Geometry check sheet. Reference: the model listing, model coordinates, mm. Give positions to 0.01 mm unless a question says otherwise; leave off trailing zeros. Write each loop counter-clockwise with the first axis right and the second up, starting at its lowest first coordinate (ties: lowest second). Pieces come first, ordered by that corner, then holes. Notation, with made-up numbers: (87.25, 33.5) -> (104.25, 33.5) arc R32 ccw to (104.25, 67.5) -> close; hole circle Ø11 at (46.5, -3). An arc over 180 degrees is marked (long way). One line per item, written item: value.
Autodesk Inventor part; units mm, degrees
ref_plane "YZ Plane" through (0, 0, 0) normal (1, 0, 0) x (0, 1, 0)
ref_plane "XZ Plane" through (0, 0, 0) normal (0, 1, 0) x (-1, 0, 0)
ref_plane "XY Plane" through (0, 0, 0) normal (0, 0, 1) x (1, 0, 0)
sketch "Sketch1" plane through (0, 0, 0) normal (0, 1, 0) x (-1, 0, 0)
  line L0 (0, 0) -> (25.4, 0)
  line L1 (25.4, 0) -> (25.4, -76.2)
  line L2 (25.4, -76.2) -> (0, -76.2)
  line L3 (0, -76.2) -> (0, 0)
  dimension "d0" = 25.4
  dimension "d1" = 76.2
extrude "Extrusion1" add sketch "Sketch1" along normal blind 3.175
sketch "Sketch2" plane through (0, 3.175, 0) normal (0, 1, 0) x (1, 0, 0)
  line L0 (-25.4, 76.2) -> (-25.4, 0)
  line L1 (0, 76.2) -> (-25.4, 76.2)
  line L2 (-25.4, 0) -> (0, 76.2)
  line L3 (0, 76.2) -> (-25.4, 76.2)
  line L4 (-25.4, 76.2) -> (0, 0)
  line L5 (0, 0) -> (-12.7, 38.1)
  line L6 (-25.4, 0) -> (0, 0)
  line L7 (-12.7, 0) -> (-12.7, 76.2)
  circle A0 centre (-12.7, 38.1) radius 3.175
  line L8 (-12.7, 38.1) -> (-12.7, 0)
  circle A1 centre (-12.7, 19.05) radius 3.175
  line L9 (-12.7, 38.1) -> (-12.7, 76.2)
  circle A2 centre (-12.7, 57.15) radius 3.175
  dimension "d4" = 6.35
  dimension "d5" = 6.35
  dimension "d6" = 6.35
extrude "Extrusion2" cut sketch "Sketch2" against normal blind 3.175 contours A0 L7 L4 | L4 L2 A0 | L2 L7 A0 | A2 L7 | L7 A2 | L7 A0 L2 | L2 A0 L4 | L4 A0 L7 | A1 L7 | L7 A1
fillet "Fillet1" radius 12.7 4 edges at (0, 1.5875, 0) (-25.4, 1.5875, 0) (0, 1.5875, -76.2) (-25.4, 1.5875, -76.2)
fillet "Fillet2" radius 0.3175 3 edges at (-15.875, 3.175, -57.15) (-15.875, 3.175, -38.1) (-15.875, 3.175, -19.05)
sketch "Sketch3" plane through (0, 3.175, 0) normal (0, 1, 0) x (1, 0, 0)
  circle A0 centre (-12.7, 57.15) radius 3.175
  circle A1 centre (-12.7, 57.15) radius 6.35
  point P0 (0, 0)
  dimension "d11" = 12.7
extrude "Extrusion3" add sketch "Sketch3" along normal blind 3.175
sketch "Sketch4" plane through (-12.7, 6.35, -57.15) normal (0, 1, 0) x (1, 0, 0)
  circle A0 centre (0, 0) radius 6.35
  circle A1 centre (0, 0) radius 3.175
  point P0 (12.7, -57.15)
extrude "Extrusion4" add sketch "Sketch4" against normal through all
fillet "Fillet3" radius 0.3175 1 edges at (-15.875, 6.35, -57.15)
sketch "Sketch5" plane through (0, 0, 0) normal (0, -1, 0) x (1, 0, 0)
  circle A0 centre (-12.7, -38.1) radius 3.175
  circle A1 centre (-12.7, -19.05) radius 3.175
  arc A2 (-25.4, -63.5) -> (0, -63.5) centre (-12.7, -63.5) ccw
  line L0 (0, -12.7) -> (0, -63.5)
  arc A3 (0, -12.7) -> (-25.4, -12.7) centre (-12.7, -12.7) ccw
  line L1 (-25.4, -63.5) -> (-25.4, -12.7)
  circle A4 centre (-12.7, -57.15) radius 3.175
  point P0 (0, 0)
extrude "Extrusion5" add sketch "Sketch5" along normal blind 3.175
properties part number "Board"
1) Sectioned sample at B-B on y = 0.75. Give the number of separate pieces and of enclosed holes in the cut face, plus the area to 3 significant figures.
Verdict:
separate pieces: 1
enclosed holes: 3
area: 1,700 mm^2
2) Sectioned sample at D-D on y = 5. Record the cut outline in (x, z) (3 decimals).
Verdict:
outline: circle Ø12.7 at (-12.7, -57.15); hole circle Ø6.35 at (-12.7, -57.15)
3) Scan lines: probe 1 along Z at (x, y) = (-12.7, 1) (3 decimals); probe 2 along X at (y, z) = (0, -57.15) (3 decimals); probe 3 along Z at (x, y) = (-12.7, 4) (3 decimals). Record each from-to range of solid material in increasing order.
Verdict:
probe 1: -76.2 to -60.325, -53.975 to -41.275, -34.925 to -22.225, -15.875 to 0
probe 2: -25.4 to -15.875, -9.525 to 0
probe 3: -63.5 to -60.325, -53.975 to -50.8
4) Depth check by flat-ended pin: pin 1 Ø2 at (x, y) = (-21.5, 3.5) entering from -Z; pin 2 Ø4 at (x, z) = (-12.7, -57.15) entering from +Y; pin 3 Ø3 at (x, y) = (-16, -0.5) entering from -Z; pin 4 Ø3 at (x, y) = (-18, 2.5) entering from -Z. Enter the tip coordinate at first touch or a pass-through.
Verdict:
pin 1: z = -73.48
pin 2: through
pin 3: z = -76.07
pin 4: z = -75.62
5) Sectioned sample at A-A on z = -19.05. Record the cut outline in (x, y) (1 decimal).
Verdict:
outline: (-25.4, -3.2) -> (-15.9, -3.2) -> (-15.9, 2.9) arc R0.3 ccw to (-16.2, 3.2) -> (-25.4, 3.2) -> close; (-9.5, -3.2) -> (0, -3.2) -> (0, 3.2) -> (-9.2, 3.2) arc R0.3 ccw to (-9.5, 2.9) -> close
6) Mould release check, pull along Y, two halves, no side actions. Record for faces 1 (the flat face through (-19, -3.175, -38)), 2 (the flat face through (-7, 3.175, -38)), 3 (the cylindrical face through (-21.58, 1.61, -72.58)): released by +Y, released by -Y, zero draft, split by the parting line, or undercut.
Verdict:
face 1: released by -Y
face 2: released by +Y
face 3: zero draft
